Model file for the job. Use its own axes, mm. A direction names the side the tool comes from. Give positions to 0.01 mm unless a question says otherwise; leave off trailing zeros. Loops run counter-clockwise (first coordinate to the right, second up) from the corner with the lowest first, then second, coordinate; pieces in that order, holes last. Notation, with made-up numbers: (31, 53) - (40, 53) arc R5 ccw to (40, 61) - close; hole circle Ø1 at (-35, 69). An arc over 180 degrees is marked (long way). Answer as CSV lines item,"result". Start each with the question number.
Item 1: Tool access for faces 4 (the flat face through (1.5, 0.9, 1.5)), 5 (the flat face through (3, 0, 4.8)), 6 (the flat face through (0, 0, 12)): list every direction of +Z, -Z, +X, -X, +Y, -Y with a clear straight run to the whole face (end or side of a thin tool).
Item 2: Saw through at A-A on z = 2. Give the cut face in (x, y), plus the area to 3 significant figures.
Item 3: Saw through at C-C on z = 7.25. Give the cut face in (x, y).
Item 4: Saw through at B-B on x = 0. Give the cut face in (y, z).
Item 5: Drill centre lines: L1, parallel to Y at x = 0, z = 0.5; L2, parallel to Z at x = -2.25, y = 3.25; L3, parallel to Z at x = -2.5, y = -0.25. Where is each one in solid material? Low to high. Write a range as from..to.
Item 6: Pull direction Y, two halves, no side cores. Call faces 1 (the cylindrical face through (0, -2, 8)), 2 (the flat face through (2, -2, 0)), 3 (the cylindrical face through (-1.655, -0.934, 0.143)): pulls with the +Y half, pulls with the -Y half, needs draft (parallel to the pull), parting line crosses it, or undercut.
Item 7: Pin check, flat tips, straight feed: pin 1 (3 mm diameter, centred on x = -4.5, y = -1, fed in from -Z); pin 2 (5 mm diameter, centred on x = 3, z = 9.5, fed in from -Y); pin 3 (5 mm diameter, centred on y = 4, z = 4, fed in from +X); pin 4 (2 mm diameter, centred on y = 4, z = 8, fed in from +X). Stop position of each tip, or through.
from build123d import *

# Parameters (mm, degrees)
SKETCH1_R           = 3.5
BOSS_EXTRUDE1_DEPTH = 4
SKETCH2_R           = 2
BOSS_EXTRUDE2_DEPTH = 8
CUT_EXTRUDE1_DEPTH  = 2.5
FILLET1_R           = 0.5
CHAMFER1_SIZE       = 0.2
SKETCH4_R           = 6
BOSS_EXTRUDE3_DEPTH = 0.8
FILLET2_R           = 0.1


with BuildPart() as part:
    # Sketch1 → Boss-Extrude1 (new body)
    with BuildSketch(Plane.XY):
        Circle(SKETCH1_R)
    extrude(amount=BOSS_EXTRUDE1_DEPTH)

    # Sketch2 → Boss-Extrude2 (add)
    with BuildSketch(Plane.XY.offset(4)):
        Circle(SKETCH2_R)
    extrude(amount=BOSS_EXTRUDE2_DEPTH)

    # Sketch3 → Cut-Extrude1 (cut)
    with BuildSketch(Plane(origin=(0, 0, 0), x_dir=(-1, 0, 0), z_dir=(0, 0, -1))):
        Polygon((2.020725942, 0), (1.010362971, 1.75), (-1.010362971, 1.75), (-2.020725942, 0), (-1.010362971, -1.75), (1.010362971, -1.75), align=None)
    extrude(amount=-CUT_EXTRUDE1_DEPTH, mode=Mode.SUBTRACT)

    # Fillet1
    fillet1_edges = [part.edges().sort_by_distance(p)[0] for p in [
        (-1.515544457, -0.875, 0),
        (-1.515544457, 0.875, 0),
        (0, 1.75, 0),
        (1.515544457, 0.875, 0),
        (1.515544457, -0.875, 0),
        (0, -1.75, 0),
        (-3.5, 0, 0),
        (-3.5, 0, 4),
        (-2, 0, 4),
    ]]
    fillet(fillet1_edges, radius=FILLET1_R)

    # Chamfer1
    chamfer1_edges = [part.edges().sort_by_distance(p)[0] for p in [
        (-2, 0, 12),
    ]]
    chamfer(chamfer1_edges, length=CHAMFER1_SIZE)

    # Sketch4 → Boss-Extrude3 (add)
    with BuildSketch(Plane.XY.offset(4)):
        Circle(SKETCH4_R)
    extrude(amount=BOSS_EXTRUDE3_DEPTH)

    # Fillet2
    fillet2_edges = [part.edges().sort_by_distance(p)[0] for p in [
        (-6, 0, 4),
        (-6, 0, 4.8),
    ]]
    fillet(fillet2_edges, radius=FILLET2_R)


solid = part.part
Responses:
1,face 4,"-Z"
1,face 5,"+Z"
1,face 6,"+Z, +X, -X, +Y, -Y"
2,outline,"circle Ø7 at (0, 0); hole (-2.02, 0) - (-1.01, -1.75) - (1.01, -1.75) - (2.02, 0) - (1.01, 1.75) - (-1.01, 1.75) - close"
2,area,"27.9 mm2"
3,outline,"circle Ø4 at (0, 0)"
4,outline,"(-6, 4.1) arc R0.1 ccw to (-5.9, 4) - (-3, 4) arc R0.5 ccw to (-3.5, 3.5) - (-3.5, 0.5) arc R0.5 ccw to (-3, 0) - (-2.25, 0) arc R0.5 ccw to (-1.75, 0.5) - (-1.75, 2.5) - (1.75, 2.5) - (1.75, 0.5) arc R0.5 ccw to (2.25, 0) - (3, 0) arc R0.5 ccw to (3.5, 0.5) - (3.5, 3.5) arc R0.5 ccw to (3, 4) - (5.9, 4) arc R0.1 ccw to (6, 4.1) - (6, 4.7) arc R0.1 ccw to (5.9, 4.8) - (2, 4.8) - (2, 11.8) - (1.8, 12) - (-1.8, 12) - (-2, 11.8) - (-2, 4.8) - (-5.9, 4.8) arc R0.1 ccw to (-6, 4.7) - close"
5,L1,"-3.5..-1.75, 1.75..3.5"
5,L2,"4..4.8"
5,L3,"0..4.8"
6,face 1,"parting line crosses it"
6,face 2,"needs draft"
6,face 3,"undercut"
7,pin 1,"z = 0.01"
7,pin 2,"y = -1.94"
7,pin 3,"x = 5.81"
7,pin 4,"through"
